Build history of the part. All positions in model axes, mm. Give positions to 0.01 mm unless a question says otherwise; leave off trailing zeros. Order: outer loops, then holes, each group sorted by start corner. A loop starts at its lowest first (then second) coordinate and runs counter-clockwise, first axis right, second up. Notation, with made-up numbers: M 82.5,55 L 92.5,55 A21 ccw 92.5,78 Z; hole C 29,74.25 d7. An arc over 180 degrees is marked long. One line per item, written item: value. Start each with the question number.
from build123d import *

# Parameters (mm, degrees)
SKETCH1_R           = 17.5
BOSS_EXTRUDE1_DEPTH = 1.6
CUT_EXTRUDE1_DEPTH  = 25.800403223
SKETCH4_R           = 1.25
CUT_EXTRUDE2_DEPTH  = 25.800403223


with BuildPart() as part:
    # Sketch1 → Boss-Extrude1 (new body)
    with BuildSketch(Plane(origin=(0, 0, -930.4), x_dir=(-1, 0, 0), z_dir=(0, 0, -1))):
        Circle(SKETCH1_R)
    extrude(amount=BOSS_EXTRUDE1_DEPTH)

    # Sketch2 → Cut-Extrude1 (cut, through all)
    with BuildSketch(Plane(origin=(0, 0, -932), x_dir=(-1, 0, 0), z_dir=(0, 0, -1))):
        with BuildLine():
            Line((-2.378923436, -16.893881238), (-2.424885778, -17.331183715))
            ThreePointArc((-2.424885778, -17.331183715), (-1.829248107, -17.404133169), (-1.231459504, -17.456617871))
            Line((-1.231459504, -17.456617871), (-1.185497161, -17.019315394))
            ThreePointArc((-1.185497161, -17.019315394), (-1.719493221, -16.359885179), (-2.378923436, -16.893881238))
        make_face()
        with BuildLine():
            ThreePointArc((1.231459504, -17.456617871), (1.829248107, -17.404133169), (2.424885778, -17.331183715))
            Line((2.424885778, -17.331183715), (2.378923436, -16.893881238))
            ThreePointArc((2.378923436, -16.893881238), (1.719493221, -16.359885179), (1.185497161, -17.019315394))
            Line((1.185497161, -17.019315394), (1.231459504, -17.456617871))
        make_face()
    extrude(amount=-CUT_EXTRUDE1_DEPTH, mode=Mode.SUBTRACT)

    # Sketch4 → Cut-Extrude2 (cut, through all)
    with BuildSketch(Plane.XY.offset(-930.4)):
        with Locations((0, 7.5)):
            Circle(SKETCH4_R)
        with Locations((0, 4)):
            Circle(SKETCH4_R)
        with Locations((0, 0.5)):
            Circle(SKETCH4_R)
        with Locations((-3.5, -6)):
            Circle(SKETCH4_R)
        with Locations((0, -6)):
            Circle(SKETCH4_R)
        with Locations((3.5, -6)):
            Circle(SKETCH4_R)
    extrude(amount=-CUT_EXTRUDE2_DEPTH, mode=Mode.SUBTRACT)


solid = part.part
1) Slice it at C-C (y = 0.5). List the corners of the cut face in (x, z).
2) Slice it at D-D (x = -3.5). List the corners of the cut face in (y, z).
3) Slice it at B-B (z = -931.5). List the corners of the cut face in (x, y), plus the area to 3 significant figures.
4) Slice it at A-A (x = 0). List the corners of the cut face in (y, z), plus the area to 3 significant figures.
5) Pull direction Y, two halves, no side cores. Call faces 1 (the flat face through (0, -4, -930.4)), 2 (the cylindrical face through (-0.27, -7.22, -931.19)), 3 (the cylindrical face through (-0.735, 17.485, -931.189)): pulls with the +Y half, pulls with the -Y half, needs draft (parallel to the pull), parting line crosses it, or undercut.
6) Drill centre lines: line 1 (Y direction, x = 0, z = -931.05); line 2 (Y direction, x = -3.5, z = -931.7); line 3 (X direction, y = 11.5, z = -931.4). Where is each one in solid material? Low to high.
Results list:
1. outline: M -17.49,-932 L -1.25,-932 L -1.25,-930.4 L -17.49,-930.4 Z; M 1.25,-932 L 17.49,-932 L 17.49,-930.4 L 1.25,-930.4 Z
2. outline: M -17.15,-932 L -7.25,-932 L -7.25,-930.4 L -17.15,-930.4 Z; M -4.75,-932 L 17.15,-932 L 17.15,-930.4 L -4.75,-930.4 Z
3. outline: M -2.42,-17.33 L -2.38,-16.89 A0.6 cw -1.19,-17.02 L -1.23,-17.46 A17.5 ccw 1.23,-17.46 L 1.19,-17.02 A0.6 cw 2.38,-16.89 L 2.42,-17.33 A17.5 ccw long Z; hole C -3.5,-6 d2.5; hole C 0,-6 d2.5; hole C 0,0.5 d2.5; hole C 0,4 d2.5; hole C 0,7.5 d2.5; hole C 3.5,-6 d2.5
3. area: 930 mm²
4. outline: M -17.5,-932 L -7.25,-932 L -7.25,-930.4 L -17.5,-930.4 Z; M -4.75,-932 L -0.75,-932 L -0.75,-930.4 L -4.75,-930.4 Z; M 1.75,-932 L 2.75,-932 L 2.75,-930.4 L 1.75,-930.4 Z; M 5.25,-932 L 6.25,-932 L 6.25,-930.4 L 5.25,-930.4 Z; M 8.75,-932 L 17.5,-932 L 17.5,-930.4 L 8.75,-930.4 Z
4. area: 40.0 mm²
5. face 1: needs draft
5. face 2: undercut
5. face 3: parting line crosses it
6. line 1: y = -17.5 to -7.25, -4.75 to -0.75, 1.75 to 2.75, 5.25 to 6.25, 8.75 to 17.5
6. line 2: y = -17.15 to -7.25, -4.75 to 17.15
6. line 3: x = -13.19 to 13.19
